Autodesk Inventor part; units mm, degrees
ref_plane "YZ Plane" through (0, 0, 0) normal (1, 0, 0) x (0, 1, 0)
ref_plane "XZ Plane" through (0, 0, 0) normal (0, 1, 0) x (-1, 0, 0)
ref_plane "XY Plane" through (0, 0, 0) normal (0, 0, 1) x (1, 0, 0)
sketch "Sketch1" plane through (0, 0, 0) normal (0, 0, 1) x (1, 0, 0)
  line L0 (-5, -18.8059) -> (-5, -60.8059)
  line L1 (-5, -60.8059) -> (30, -60.8059)
  line L2 (30, -60.8059) -> (30, -18.8059)
  circle A0 centre (2, -26.8059) radius 2
  circle A1 centre (23, -26.8059) radius 2
  circle A2 centre (2, -26.8059) radius 4
  circle A3 centre (23, -26.8059) radius 4
  line L3 (30, -18.8059) -> (-5, -18.8059)
  point P0 (0, -10)
  dimension "d17" = 35
  dimension "d19" = 4
  dimension "d20" = 4
  dimension "d22" = 8
  dimension "d23" = 8
  dimension "d29" = 7
  dimension "d60" = 42
  dimension "d61" = 8
  dimension "d62" = 8
  dimension "d63" = 21
extrude "Extrusion2" add sketch "Sketch1" along normal blind 10 contours L3 L2 L1 L0 | A2 | A3
sketch "Sketch4" plane through (-5, -60.8059, 0) normal (0, -1, 0) x (1, 0, 0)
  circle A0 centre (17.5, 5) radius 3
  line L0 (35, 0) -> (35, 10)
  line L1 (0, 10) -> (35, 10)
  dimension "d48" = 6
  dimension "d49" = 17.5
  dimension "d50" = 5
extrude "Extrusion5" cut sketch "Sketch4" against normal blind 30
thread "Thread2"
chamfer "Chaflán1" distance 2.5 angle 45 2 edges at (0, -26.8059, 10) (21, -26.8059, 10)
equation "\"d61\" = d62"
properties part number "Soporte para Patas Regulables" material "Aluminum 6061"
Build history of the part. All positions in model axes, mm. A direction names the side the tool comes from. Round coordinates to 2 decimals unless told otherwise and drop trailing zeros. Write each loop counter-clockwise with the first axis right and the second up, starting at its lowest first coordinate (ties: lowest second). Pieces come first, ordered by that corner, then holes. Notation, with made-up numbers: M -35,28 L -23,28 A26 ccw -23,67 Z; hole C 88.5,22 d9. An arc over 180 degrees is marked long. Answer as a JSON object with one key per item and string values. Group by question number.
(1) Cut at D-D (x = 12.5). Give the cut face in (y, z).
(2) Which spindle directions (+Z, -Z, +X, -X, +Y, -Y) get a long thin tool onto all of the face, cutting with end or side? Do faces 1 (the flat face through (12.3, -60.806, 1.6)), 2 (the flat face through (12, -30.806, 5)). Say none if no direction does.
(3) Cut at C-C (z = 3.75). Give the cut face in (x, y).
(4) Mould opens along X. For faces 3 (the cylindrical face through (1.74, -28.79, 3.7)), 4 (the flat face through (-5, -40, 5)), 5 (the flat face through (12, -40, 0)), 6 (the flat face through (30, -40, 5)) say: pulls with the +X half, pulls with the -X half, needs draft (parallel to the pull), parting line crosses it, or undercut.
(5) Cut at B-B (y = -35). Give the cut face in (x, z), and give its area (3 significant figures).
(6) Drill centre lines: L1, parallel to X at y = -28.5, z = 5; L2, parallel to X at y = -56.5, z = 4.75; L3, parallel to Y at x = 23, z = 6. Where is each one in solid material? Low to high.
(7) Cut at A-A (x = 23). Give the cut face in (y, z).
Responses:
{
 "1": {"outline": "M -60.81,0 L -18.81,0 L -18.81,10 L -60.81,10 L -60.81,8 L -30.81,8 L -30.81,2 L -60.81,2 Z"},
 "2": {"face 1": "+Z, -Z, +X, -X, -Y", "face 2": "-Y"},
 "3": {"outline": "M -5,-60.81 L 9.77,-60.81 L 9.77,-30.81 L 15.23,-30.81 L 15.23,-60.81 L 30,-60.81 L 30,-18.81 L -5,-18.81 Z; hole C 2,-26.81 d4; hole C 23,-26.81 d4"},
 "4": {"face 3": "undercut", "face 4": "pulls with the -X half", "face 5": "needs draft", "face 6": "pulls with the +X half"},
 "5": {"outline": "M -5,0 L 30,0 L 30,10 L -5,10 Z; hole C 12.5,5 d6", "area": "322 mm2"},
 "6": {"L1": "x = -5 to 0.94, 3.06 to 21.94, 24.06 to 30", "L2": "x = -5 to 9.51, 15.49 to 30", "L3": "y = -60.81 to -28.81, -24.81 to -18.81"},
 "7": {"outline": "M -60.81,0 L -28.81,0 L -28.81,7.5 L -31.31,10 L -60.81,10 Z; M -24.81,0 L -18.81,0 L -18.81,10 L -22.31,10 L -24.81,7.5 Z"}
}
